Work out the finished part from the listing and answer in its coordinate system (mm). Round coordinates to 2 decimals unless told otherwise and drop trailing zeros. Loops run counter-clockwise (first coordinate to the right, second up) from the corner with the lowest first, then second, coordinate; pieces in that order, holes last. Notation, with made-up numbers: (-9.5, 25.25) - (6.5, 25.25) arc R20 ccw to (6.5, 40.25) - close; hole circle Ø7 at (-25, 50). An arc over 180 degrees is marked (long way). Answer as CSV lines item,"result". Start each with the question number.
Q1. Straight lines are drawn through the part: L1, parallel to X at y = -9, z = 54; L2, parallel to X at y = 9, z = 77.5; L3, parallel to Y at x = 0, z = 40 (3 decimals). For each, find the intervals that lie inside material, in ascending order. Write a range as [from, to].
Q2. Section A-A on x = 0 is taken. Write down the section's boundary in (y, z).
Q3. The mould has two halves that part along X. Classify faces 1 (the face through (-1.323, 10.074, 45.072)), 2 (the face through (-2.75, -12.4, 76.02)), 3 (the face through (-6, 9, 88.9)): +X half, -X half, draft (parallel to the pull), parting line (faces both ways), or undercut.
Q4. Section C-C on z = 79 is taken. Write down the section's boundary in (x, y), then the cut area to 3 significant figures.
Q5. Each of these flat-tipped pins is pushed along its axis until it touches: pin 1 Ø1 at (y, z) = (10.5, 14) entering from +X; pin 2 Ø1 at (y, z) = (-7, 53) entering from -X; pin 3 Ø8 at (x, z) = (6, 48.5) entering from +Y; pin 4 Ø1.5 at (x, y) = (-5.5, -12) entering from -Z. Where does it stop, or does it pass through?
Q6. Section B-B on z = 18.5 is taken. Write down the section's boundary in (x, y), then the cut area to 3 significant figures.
```python
from build123d import *

# Parameters (mm, degrees)
F0_R      = 15.24
F1_DEPTH  = 12.7
F3_R      = 12.7
F1_FACE_R = 15.24
F5_R      = 12.7
F6_DEPTH  = 25.4
F7_R      = 10.16
F8_DEPTH  = 88.901


with BuildPart() as f1:
    # F0 (on Top) → F1 (new body)
    with BuildSketch(Plane.XY):
        Circle(F0_R)
    extrude(amount=F1_DEPTH)

    # F3 (on offset) → F4 section 0
    with BuildSketch(Plane.XY.offset(63.5)):
        Circle(F3_R)
    # F1_face (on face) → F4 section 1
    with BuildSketch(Plane.XY.offset(12.7)):
        Circle(F1_FACE_R)
    loft()

    # F5 (on face) → F6 (join)
    with BuildSketch(Plane.XY.offset(63.5)):
        Circle(F5_R)
    extrude(amount=F6_DEPTH)

    # F7 (on face) → F8 (cut, through all)
    with BuildSketch(Plane.XY.offset(88.9)):
        Circle(F7_R)
    extrude(amount=-F8_DEPTH, mode=Mode.SUBTRACT)


solid = f1.part
```
Findings:
1,L1,"x = [-9.62, -4.71], [4.71, 9.62]"
1,L2,"x = [-8.96, -4.71], [4.71, 8.96]"
1,L3,"y = [-13.875, -10.16], [10.16, 13.875]"
2,outline,"(-15.24, 0) - (-10.16, 0) - (-10.16, 88.9) - (-12.7, 88.9) - (-12.7, 63.5) - (-15.24, 12.7) - close; (10.16, 0) - (15.24, 0) - (15.24, 12.7) - (12.7, 63.5) - (12.7, 88.9) - (10.16, 88.9) - close"
3,face 1,"undercut"
3,face 2,"parting line"
3,face 3,"draft"
4,outline,"circle Ø25.4 at (0, 0); hole circle Ø20.32 at (0, 0)"
4,area,"182 mm^2"
5,pin 1,"stops at x = 11.42"
5,pin 2,"stops at x = -11.52"
5,pin 3,"stops at y = 13.33"
5,pin 4,"stops at z = 0"
6,outline,"circle Ø29.9 at (0, 0); hole circle Ø20.32 at (0, 0)"
6,area,"378 mm^2"
